```python
from build123d import *

# Parameters (mm, degrees)
CORTAR_EXTRUIR1_DEPTH = 35
CROQUIS3_W            = 5.6
CROQUIS3_H            = 2.5
CORTAR_EXTRUIR2_DEPTH = 35
CROQUIS4_R            = 1.5
CORTAR_EXTRUIR3_DEPTH = 12


with BuildPart() as part:
    # Croquis1 → Revolución1 (revolve)
    with BuildSketch(Plane(origin=(0, 0, 0), x_dir=(0, 0, -1), z_dir=(1, 0, 0))):
        Polygon((-24, 7.5), (-24, 11), (-22.5, 11), (-22.5, 9.5), (16.5, 9.5), (16.5, 11), (18, 11), (18, 8), (10, 8), (10, 0), (0, 0), (0, 7.5), align=None)
    revolve(axis=Axis((0, 0, 0), (0, 0, 1)))

    # Croquis2 → Cortar-Extruir1 (cut, through all)
    with BuildSketch(Plane(origin=(0, 0, -10), x_dir=(-1, 0, 0), z_dir=(0, 0, -1))):
        with BuildLine():
            Line((-1.17260394, 1.125), (1.17260394, 1.125))
            ThreePointArc((1.17260394, 1.125), (0, -1.625), (-1.17260394, 1.125))
        make_face()
    extrude(amount=-CORTAR_EXTRUIR1_DEPTH, mode=Mode.SUBTRACT)

    # Croquis3 → Cortar-Extruir2 (cut, through all)
    with BuildSketch(Plane(origin=(0, 0, -10), x_dir=(-1, 0, 0), z_dir=(0, 0, -1))):
        with Locations((0, 3.375)):
            Rectangle(CROQUIS3_W, CROQUIS3_H)
    extrude(amount=-CORTAR_EXTRUIR2_DEPTH, mode=Mode.SUBTRACT)

    # Croquis4 → Cortar-Extruir3 (cut, through all)
    with BuildSketch(Plane(origin=(0, 0, 0), x_dir=(1, 0, 0), z_dir=(0, 1, 0))):
        with Locations((0, 5)):
            Circle(CROQUIS4_R)
    extrude(amount=CORTAR_EXTRUIR3_DEPTH, mode=Mode.SUBTRACT)


solid = part.part
```
Can you work these out from the model? Positions are in its coordinate system, mm. A direction names the side the tool comes from. Give positions to 0.01 mm unless a question says otherwise; leave off trailing zeros. Loops run counter-clockwise (first coordinate to the right, second up) from the corner with the lowest first, then second, coordinate; pieces in that order, holes last. Notation, with made-up numbers: M 1.25,54.5 L 17.25,54.5 A8 cw 17.25,63.5 Z; hole C 42,40 d1. An arc over 180 degrees is marked long. One line per question, with ' | ' between items. Start each with the question number.
Q1. If I drill on line 1 (Y direction, x = 0, z = 10); line 2 (Y direction, x = 0, z = -8) (3 decimals), over which ranges is the centre line in solid material (lowest first)? Write a range as from..to.
Q2. For faces 5 (the flat face through (0, 1.125, -2)), 6 (the cylindrical face through (-0.33, -7.493, 12.168)), 7 (the cylindrical face through (7.81, -1.73, -13.94)), 8 (the flat face through (0, -10, 22.5)), 9 (the cylindrical face through (-1.5, 7.03, -5.07)), which set-ups out of +Z, -Z, +X, -X, +Y, -Y let a thin tool reach every point of the face, with its end or its side?
Q3. If we section it at B-B (x = -2.25): Please give me the cut outline in (y, z) (3 decimals).
Q4. If we section it at D-D (z = -13.5): Please give me the cut outline in (x, y).
Q5. For pin 1 Ø1 at (y, z) = (-4.5, -11) entering from +X; pin 2 Ø1.2 at (y, z) = (3.5, -5.5) entering from +X; pin 3 Ø1.8 at (x, z) = (0, -5) entering from -Y; pin 4 Ø2 at (x, y) = (0, 0) entering from -Z, each with a flat end and sliding along its axis, tell me the tip position at first contact or that it passes through.
Q6. If we section it at C-C (y = 6.75): Please give me the cut outline in (x, z), plus the area to 3 significant figures.
Q7. If we mould it in two halves opening along Z, with no side actions, what happens to faces 1 (the flat face through (-2.8, 3, -5)), 2 (the flat face through (-2, 0, 0)), 3 (the flat face through (8, -2, -18)), 4 (the cylindrical face through (1.43, 1.53, -5.45))? For each: +Z half, -Z half, draft (parallel to the pull), parting line (faces both ways), or undercut.
Q8. If we section it at A-A (y = 0): Please give me the cut outline in (x, z) (3 decimals).
Computed:
1) line 1: y = -9.5..-7.5, 7.5..9.5 | line 2: y = -9.5..-1.625, 1.125..2.125, 4.625..9.5
2) face 5: +Z, -Z | face 6: +Z | face 7: -Z | face 8: none | face 9: +Y
3) outline: M -10.767,-18 L -7.677,-18 L -7.677,-10 L 2.125,-10 L 2.125,0 L -7.155,0 L -7.155,24 L -10.767,24 L -10.767,22.5 L -9.23,22.5 L -9.23,-16.5 L -10.767,-16.5 Z; M 4.625,-10 L 7.677,-10 L 7.677,-18 L 10.767,-18 L 10.767,-16.5 L 9.23,-16.5 L 9.23,22.5 L 10.767,22.5 L 10.767,24 L 7.155,24 L 7.155,0 L 4.625,0 Z
4) outline: C 0,0 d19; hole C 0,0 d16
5) pin 1: stops at x = 8.62 | pin 2: stops at x = 9.05 | pin 3: stops at y = -9.5 | pin 4: passes through
6) outline: M -8.69,-18 L -4.29,-18 L -4.29,-10 L 4.29,-10 L 4.29,-18 L 8.69,-18 L 8.69,-16.5 L 6.68,-16.5 L 6.68,22.5 L 8.69,22.5 L 8.69,24 L 3.27,24 L 3.27,0 L -3.27,0 L -3.27,24 L -8.69,24 L -8.69,22.5 L -6.68,22.5 L -6.68,-16.5 L -8.69,-16.5 Z; hole C 0,-5 d3 | area: 341 mm²
7) face 1: draft | face 2: +Z half | face 3: -Z half | face 4: undercut
8) outline: M -11,-18 L -8,-18 L -8,-10 L -1.625,-10 L -1.625,0 L -7.5,0 L -7.5,24 L -11,24 L -11,22.5 L -9.5,22.5 L -9.5,-16.5 L -11,-16.5 Z; M 1.625,-10 L 8,-10 L 8,-18 L 11,-18 L 11,-16.5 L 9.5,-16.5 L 9.5,22.5 L 11,22.5 L 11,24 L 7.5,24 L 7.5,0 L 1.625,0 Z
